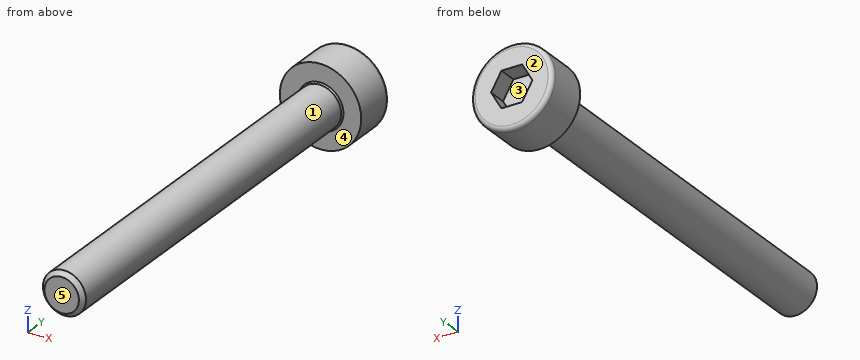
from build123d import *

# Parameters (mm, degrees)
SKETCH_1_R          = 2.84
EXTRUDE_1_DEPTH     = 3
CUT_EXTRUDE_1_DEPTH = 1.3
SKETCH_3_R          = 1.5
EXTRUDE_2_DEPTH     = 28
CHAMFER_1_SIZE      = 0.3
FILLET_1_R          = 0.3
CHAMFER_2_SIZE      = 0.1


with BuildPart() as part:
    # 草图1 → 凸台-拉伸1 (new body)
    with BuildSketch(Plane(origin=(0, 0, 0), x_dir=(1, 0, 0), z_dir=(0, 1, 0))):
        Circle(SKETCH_1_R)
    extrude(amount=EXTRUDE_1_DEPTH)

    # 草图2 → 切除-拉伸1 (cut)
    with BuildSketch(Plane(origin=(0, 3, 0), x_dir=(1, 0, 0), z_dir=(0, 1, 0))):
        Polygon((1.443375673, 0), (0.721687836, 1.25), (-0.721687836, 1.25), (-1.443375673, 0), (-0.721687836, -1.25), (0.721687836, -1.25), align=None)
    extrude(amount=-CUT_EXTRUDE_1_DEPTH, mode=Mode.SUBTRACT)

    # 草图3 → 凸台-拉伸2 (add)
    with BuildSketch(Plane.XZ):
        Circle(SKETCH_3_R)
    extrude(amount=EXTRUDE_2_DEPTH)

    # 倒角1
    chamfer_1_edges = [part.edges().sort_by_distance(p)[0] for p in [
        (-1.5, -28, 0),
    ]]
    chamfer(chamfer_1_edges, length=CHAMFER_1_SIZE)

    # 圆角1
    fillet_1_edges = [part.edges().sort_by_distance(p)[0] for p in [
        (-2.84, 3, 0),
    ]]
    fillet(fillet_1_edges, radius=FILLET_1_R)

    # 倒角2
    chamfer_2_edges = [part.edges().sort_by_distance(p)[0] for p in [
        (-1.5, 0, 0),
    ]]
    chamfer(chamfer_2_edges, length=CHAMFER_2_SIZE)


solid = part.part
Design review of the part built by this model. Coordinates are the model's own, in mm. Face numbers are marked on the shaded views. A direction names the side the tool comes from. Coordinates: 2 decimals unless noted, no trailing zeros. Order: outer loops, then holes, each group sorted by start corner. A loop starts at its lowest first (then second) coordinate and runs counter-clockwise, first axis right, second up. Notation, with made-up numbers: M 80,44 L 119,44 A16 ccw 119,69 Z; hole C 85.5,0.25 d5. An arc over 180 degrees is marked long. Use a Markdown table: item, result.
(1) For the marked faces 4 and 5, list the 3-axis set-ups (+Z, -Z, +X, -X, +Y, -Y) from which the entire face can be reached by the end or side of a thin tool; tool diameter is ignored.
Worked answers:
| item | result |
|---|---|
| face 4 | -Y |
| face 5 | +Z, -Z, +X, -X, -Y |
(2) Draft analysis for pull direction Z (two halves, no side actions). For the marked faces 1, 2 and 3, state which applies: released by +Z, released by -Z, zero draft, split by the parting line, or undercut.
Worked answers:
| item | result |
|---|---|
| face 1 | split by the parting line |
| face 2 | zero draft |
| face 3 | undercut |
(3) Wall thickness on probe 1 along Z at (x, y) = (-0.1, 1); probe 2 along Y at (x, z) = (0.1, -0.1); probe 3 along Y at (x, z) = (-0.55, -2.2): over which ranges is each line inside the solid? List them lowest first.
Worked answers:
| item | result |
|---|---|
| probe 1 | z = -2.84 to 2.84 |
| probe 2 | y = -28 to 1.7 |
| probe 3 | y = 0 to 3 |
(4) Add section A-A (x = 0). Give the boundary of the cut face in (y, z), then the cut area to 3 significant figures.
Worked answers:
| item | result |
|---|---|
| outline | M -28,-1.2 L -27.7,-1.5 L -0.1,-1.5 L 0,-1.6 L 0,-2.84 L 2.7,-2.84 A0.3 ccw 3,-2.54 L 3,-1.25 L 1.7,-1.25 L 1.7,1.25 L 3,1.25 L 3,2.54 A0.3 ccw 2.7,2.84 L 0,2.84 L 0,1.6 L -0.1,1.5 L -27.7,1.5 L -28,1.2 Z |
| area | 97.7 mm2 |
(5) Add section B-B (y = -14.5). Give the boundary of the cut face in (x, z).
Worked answers:
| item | result |
|---|---|
| outline | C 0,0 d3 |
